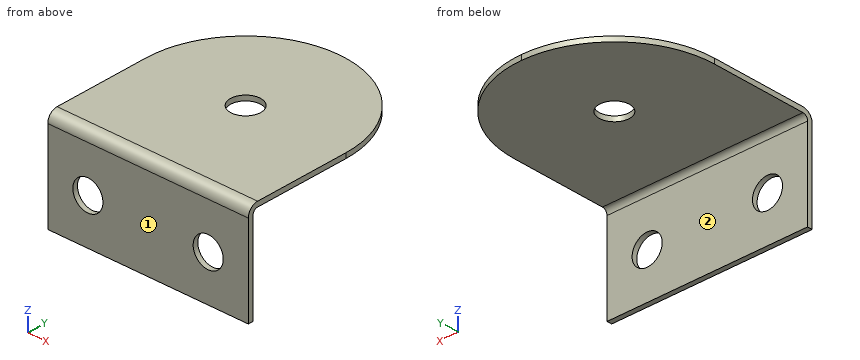
from build123d import *

# Parameters (mm, degrees)
BRIDA_BASE1_DEPTH     = 20
CROQUIS5_R            = 1.5
CORTAR_EXTRUIR1_DEPTH = 10
CROQUIS6_R            = 1.5
CORTAR_EXTRUIR2_DEPTH = 10


# Sheet-metal steps are written as plain solids
with BuildPart() as part:
    # Croquis1 → Brida base1 (new body)
    with BuildSketch(Plane(origin=(0, 0, 0), x_dir=(0, 0, -1), z_dir=(1, 0, 0))):
        with BuildLine():
            Line((0, 20.5), (0, 1))
            ThreePointArc((0, 1), (0.292893219, 0.292893219), (1, 0))
            Line((1, 0), (10, 0))
            Line((10, 0), (10, 0.5))
            Line((10, 0.5), (1, 0.5))
            ThreePointArc((1, 0.5), (0.646446609, 0.646446609), (0.5, 1))
            Line((0.5, 1), (0.5, 20.5))
            Line((0.5, 20.5), (0, 20.5))
        make_face()
    extrude(amount=BRIDA_BASE1_DEPTH)

    # Croquis5 → Cortar-Extruir1 (cut)
    with BuildSketch(Plane(origin=(0, 0.5, 0), x_dir=(1, 0, 0), z_dir=(0, 1, 0))):
        with Locations(Location((4, 5.5, 0), (0, 0, 270))):
            Circle(CROQUIS5_R)
        with Locations(Location((16, 5.5, 0), (0, 0, 270))):
            Circle(CROQUIS5_R)
    extrude(amount=-CORTAR_EXTRUIR1_DEPTH, mode=Mode.SUBTRACT)

    # Croquis6 → Cortar-Extruir2 (cut)
    with BuildSketch(Plane.XY):
        with BuildLine():
            ThreePointArc((0, 10.5), (2.928932188, 17.571067812), (10, 20.5))
            Line((10, 20.5), (0, 20.5))
            Line((0, 20.5), (0, 10.5))
        make_face()
        with BuildLine():
            ThreePointArc((10, 20.5), (17.071067812, 17.571067812), (20, 10.5))
            Line((20, 10.5), (20, 20.5))
            Line((20, 20.5), (10, 20.5))
        make_face()
        with Locations(Location((10, 10.5, 0), (0, 0, 90))):
            Circle(CROQUIS6_R)
    extrude(amount=-CORTAR_EXTRUIR2_DEPTH, mode=Mode.SUBTRACT)


solid = part.part
The listing builds one solid part. Answer for the finished solid, in the listing's coordinates (mm). Face numbers are marked on the shaded views. A direction names the side the tool comes from. Give positions to 0.01 mm unless a question says otherwise; leave off trailing zeros. Loops run counter-clockwise (first coordinate to the right, second up) from the corner with the lowest first, then second, coordinate; pieces in that order, holes last. Notation, with made-up numbers: (21, 70.5) - (61, 70.5) arc R18 ccw to (61, 104.5) - close; hole circle Ø7 at (6, -27.5). An arc over 180 degrees is marked (long way). Use one line per item in the form item = value.
1. Section A-A on z = -5.5 is taken. Give the vertices of the cut face in (x, y), then the cut area to 3 significant figures.
Calculated:
outline = (0, 0) - (2.5, 0) - (2.5, 0.5) - (0, 0.5) - close; (5.5, 0) - (14.5, 0) - (14.5, 0.5) - (5.5, 0.5) - close; (17.5, 0) - (20, 0) - (20, 0.5) - (17.5, 0.5) - close
area = 7.00 mm^2
2. Find the intervals of material crossed by line 1 along X through (y, z) = (0.35, -5.5); line 2 along X through (y, z) = (10.5, -0.2); line 3 along Y through (x, z) = (18.5, -2), in increasing order. Write a range as [from, to].
Calculated:
line_1 = [0, 2.5], [5.5, 14.5], [17.5, 20]
line_2 = [0, 8.5], [11.5, 20]
line_3 = [0, 0.5]
3. Section C-C on y = 8.25 is taken. Give the vertices of the cut face in (x, z).
Calculated:
outline = (0, -0.5) - (20, -0.5) - (20, 0) - (0, 0) - close
4. Which of the six approach directions +Z, -Z, +X, -X, +Y, -Y give full straight-line access (tool end or side, diameter ignored) to the marked faces 1 and 2?
Calculated:
face_1 = +Z, -Z, +X, -X, -Y
face_2 = -Z, +X, -X, +Y
5. Section D-D on z = -8 is taken. Give the vertices of the cut face in (x, y), then the cut area to 3 significant figures.
Calculated:
outline = (0, 0) - (20, 0) - (20, 0.5) - (0, 0.5) - close
area = 10.0 mm^2
6. Section B-B on x = 16 is taken. Give the vertices of the cut face in (y, z), then the cut area to 3 significant figures.
Calculated:
outline = (0, -10) - (0.5, -10) - (0.5, -7) - (0, -7) - close; (0, -4) - (0.5, -4) - (0.5, -1) arc R0.5 cw to (1, -0.5) - (18.5, -0.5) - (18.5, 0) - (1, 0) arc R1 ccw to (0, -1) - close
area = 12.3 mm^2
7. Given pin 1 Ø5 at (x, z) = (16, -5.5) entering from +Y; pin 2 Ø5 at (x, y) = (9.5, 18) entering from -Z, each flat-ended and moving along its own axis, determine where each tip first touches the part or whether it passes through.
Calculated:
pin_1 = 0.5
pin_2 = -0.5
